Input: part model. Units: mm. Frame: model coordinates. A direction names the side the tool comes from. Coordinates: 2 decimals unless noted, no trailing zeros. Write each loop counter-clockwise with the first axis right and the second up, starting at its lowest first coordinate (ties: lowest second). Pieces come first, ordered by that corner, then holes. Notation, with made-up numbers: (73.25, 71.5) - (103.25, 71.5) arc R9 ccw to (103.25, 84.5) - close; hole circle Ø6 at (-19.5, 41.5). An arc over 180 degrees is marked (long way). One line per question, with ' | ' between items. Start each with the question number.
1) Draft query along Y for faces 4 (the flat face through (-11, -5, 6)), 5 (the cylindrical face through (-32.69, 0.96, 1.51)), 6 (the flat face through (-17.73, -5.51, 2.96)). Return one class per face: released by +Y, released by -Y, zero draft, split by the parting line, or undercut.
2) First-contact query: P1, Ø3, axis at x = 0, y = 0, coming from the +Z side; P2, Ø1.5, axis at x = -15.5, z = 5, coming from the -Y side; P3, Ø6, axis at x = 0, y = 0, coming from the -Z side. Flat tips, straight axial feed; report the tip coordinate or a pass-through.
3) Section query A-A on x = 0. Return loops of the section in (y, z).
4) Section query D-D on x = -18. Return loops of the section in (y, z).
5) Line query: line 1 (Y direction, x = 0, z = 5.55); line 2 (Y direction, x = 0, z = 2.5); line 3 (Z direction, x = -1, y = 2.75). Output: solid intervals per line, ascending.
6) Reachability of faces 1 (the flat face through (-36, -2, 2.5)), 2 (the flat face through (-14.1, 3.7, 3)), 3 (the flat face through (-1, -1, 4.5)) from +Z, -Z, +X, -X, +Y, -Y: full face, straight path, thin tool, end or side. Return the list, or none.
7) Section query B-B on z = 1.5. Return loops of the section in (x, y).
8) Section query C-C on y = 0. Give the number of separate pieces and of enclosed holes in the cut face, and give its area (3 significant figures).
```python
from build123d import *

# Parameters (mm, degrees)
EXTRUDE_1_DEPTH      = 6
CUT_EXTRUDE_1_DEPTH  = 41.077836542
FILLET_1_R           = 1
SKETCH_7_R           = 2
CUT_EXTRUDE_2_DEPTH  = 41.077836542
SKETCH_7_4_R         = 2.5
SKETCH_7_4_R_2       = 2
CUT_EXTRUDE_4_DEPTH  = 2.5
SKETCH_7_5_R         = 3
SKETCH_7_5_R_2       = 2.5
CUT_EXTRUDE_5_DEPTH  = 0.5
CUT_EXTRUDE_9_DEPTH  = 4
SKETCH_13_R          = 1.25
CUT_EXTRUDE_10_DEPTH = 40.827540495
SKETCH_14_R          = 2.5
CUT_EXTRUDE_11_DEPTH = 1.5
CUT_EXTRUDE_START    = -2.5
SKETCH_15_R          = 2.5
CUT_EXTRUDE_13_DEPTH = 2.5
CUT_EXTRUDE_START_2  = -0.5
SKETCH_15_4_R        = 3
SKETCH_15_4_R_2      = 2.5
CUT_EXTRUDE_14_DEPTH = 0.5


with BuildPart() as part:
    # Sketch 2 → Extrude 1 (new body)
    with BuildSketch(Plane.XY):
        with BuildLine():
            Line((-35.344756781, 3.98511515), (-0.604756988, 6.99051149))
            ThreePointArc((-0.604756988, 6.99051149), (7.01662183, 0), (-0.604756988, -6.99051149))
            Line((-0.604756988, -6.99051149), (-35.344756781, -3.98511515))
            ThreePointArc((-35.344756781, -3.98511515), (-39, 0), (-35.344756781, 3.98511515))
        make_face()
    extrude(amount=EXTRUDE_1_DEPTH)

    # Sketch 6 → Cut-Extrude 1 (cut, through all)
    with BuildSketch(Plane.XY.offset(6)):
        Polygon((-30.385995652, 2.291125705), (-22.385995652, 2.983214677), (-22.385995652, -2.983214677), (-30.385995652, -2.291125705), align=None)
        Polygon((-19.385995652, 3.242748041), (-19.385995652, -3.242748041), (-8.71565209, -4.165851428), (-8.71565209, 4.165851428), align=None)
    extrude(amount=-CUT_EXTRUDE_1_DEPTH, mode=Mode.SUBTRACT)

    # Fillet 1
    fillet_1_edges = [part.edges().sort_by_distance(p)[0] for p in [
        (-30.385995652, -2.291125705, 3),
        (-30.385995652, 2.291125705, 3),
        (-22.385995652, 2.983214677, 3),
        (-22.385995652, -2.983214677, 3),
        (-8.71565209, -4.165851428, 3),
        (-19.385995652, -3.242748041, 3),
        (-19.385995652, 3.242748041, 3),
        (-8.71565209, 4.165851428, 3),
    ]]
    fillet(fillet_1_edges, radius=FILLET_1_R)

    # Sketch 7 → Cut-Extrude 2 (cut, through all)
    with BuildSketch(Plane.XY.offset(6)):
        with Locations((-35, 0)):
            Circle(SKETCH_7_R)
    extrude(amount=-CUT_EXTRUDE_2_DEPTH, mode=Mode.SUBTRACT)

    # Sketch 7_4 → Cut-Extrude 4 (cut)
    with BuildSketch(Plane.XY.offset(6)):
        with Locations((-35, 0)):
            Circle(SKETCH_7_4_R)
        with Locations((-35, 0)):
            Circle(SKETCH_7_4_R_2, mode=Mode.SUBTRACT)
    extrude(amount=-CUT_EXTRUDE_4_DEPTH, mode=Mode.SUBTRACT)

    # Sketch 7_5 → Cut-Extrude 5 (cut)
    with BuildSketch(Plane.XY.offset(6)):
        with Locations((-35, 0)):
            Circle(SKETCH_7_5_R)
        with Locations((-35, 0)):
            Circle(SKETCH_7_5_R_2, mode=Mode.SUBTRACT)
    extrude(amount=-CUT_EXTRUDE_5_DEPTH, mode=Mode.SUBTRACT)

    # Sketch 12 → Cut-Extrude 9 (cut)
    with BuildSketch(Plane(origin=(0, 0, 0), x_dir=(-1, 0, 0), z_dir=(0, 0, -1))):
        with BuildLine():
            Line((12.25, 1.984313483), (0.4375, 3.472548596))
            ThreePointArc((0.4375, 3.472548596), (-3.5, 0), (0.4375, -3.472548596))
            Line((0.4375, -3.472548596), (12.25, -1.984313483))
            ThreePointArc((12.25, -1.984313483), (14, 0), (12.25, 1.984313483))
        make_face()
    extrude(amount=-CUT_EXTRUDE_9_DEPTH, mode=Mode.SUBTRACT)

    # Sketch 13 → Cut-Extrude 10 (cut, through all)
    with BuildSketch(Plane(origin=(0, 0, 4), x_dir=(-1, 0, 0), z_dir=(0, 0, -1))):
        Circle(SKETCH_13_R)
    extrude(amount=-CUT_EXTRUDE_10_DEPTH, mode=Mode.SUBTRACT)

    # Sketch 14 → Cut-Extrude 11 (cut)
    with BuildSketch(Plane.XY.offset(6)):
        Circle(SKETCH_14_R)
    extrude(amount=-CUT_EXTRUDE_11_DEPTH, mode=Mode.SUBTRACT)

    # Sketch 15 → Cut-Extrude 13 (cut)
    with BuildSketch(Plane(origin=(0, 0, 0), x_dir=(-1, 0, 0), z_dir=(0, 0, -1)).offset(CUT_EXTRUDE_START)):
        with Locations(Location((35, 0, 0), (0, 0, 180))):
            Circle(SKETCH_15_R)
    extrude(amount=CUT_EXTRUDE_13_DEPTH, mode=Mode.SUBTRACT)

    # Sketch 15_4 → Cut-Extrude 14 (cut)
    with BuildSketch(Plane(origin=(0, 0, 0), x_dir=(-1, 0, 0), z_dir=(0, 0, -1)).offset(CUT_EXTRUDE_START_2)):
        with Locations(Location((35, 0, 0), (0, 0, 180))):
            Circle(SKETCH_15_4_R)
        with Locations((35, 0)):
            Circle(SKETCH_15_4_R_2, mode=Mode.SUBTRACT)
    extrude(amount=CUT_EXTRUDE_14_DEPTH, mode=Mode.SUBTRACT)


solid = part.part
```
Answer key:
1) face 4: zero draft | face 5: undercut | face 6: released by -Y
2) P1: z = 4.5 | P2: y = -5.77 | P3: z = 4
3) outline: (-7.02, 0) - (-3.5, 0) - (-3.5, 4) - (-1.25, 4) - (-1.25, 4.5) - (-2.5, 4.5) - (-2.5, 6) - (-7.02, 6) - close; (1.25, 4) - (3.5, 4) - (3.5, 0) - (7.02, 0) - (7.02, 6) - (2.5, 6) - (2.5, 4.5) - (1.25, 4.5) - close
4) outline: (-5.49, 0) - (-3.36, 0) - (-3.36, 6) - (-5.49, 6) - close; (3.36, 0) - (5.49, 0) - (5.49, 6) - (3.36, 6) - close
5) line 1: -7.02 to -2.5, 2.5 to 7.02 | line 2: -7.02 to -3.5, 3.5 to 7.02 | line 3: 4 to 6
6) face 1: -Z | face 2: +Z, -Z | face 3: +Z
7) outline: (-35.34, -3.99) - (-0.6, -6.99) arc R7.02 ccw (long way) to (-0.6, 6.99) - (-35.34, 3.99) arc R4 ccw to start; hole circle Ø5 at (-35, 0); hole (-30.39, -1.37) arc R1 ccw to (-29.47, -2.37) - (-23.47, -2.89) arc R1 ccw to (-22.39, -1.89) - (-22.39, 1.89) arc R1 ccw to (-23.47, 2.89) - (-29.47, 2.37) arc R1 ccw to (-30.39, 1.37) - close; hole (-19.39, -2.33) arc R1 ccw to (-18.47, -3.32) - (-9.8, -4.07) arc R1 ccw to (-8.72, -3.08) - (-8.72, -2.43) - (-0.44, -3.47) arc R3.5 ccw (long way) to (-0.44, 3.47) - (-8.72, 2.43) - (-8.72, 3.08) arc R1 ccw to (-9.8, 4.07) - (-18.47, 3.32) arc R1 ccw to (-19.39, 2.33) - close
8) separate pieces: 5 | enclosed holes: 0 | area: 76.5 mm²
